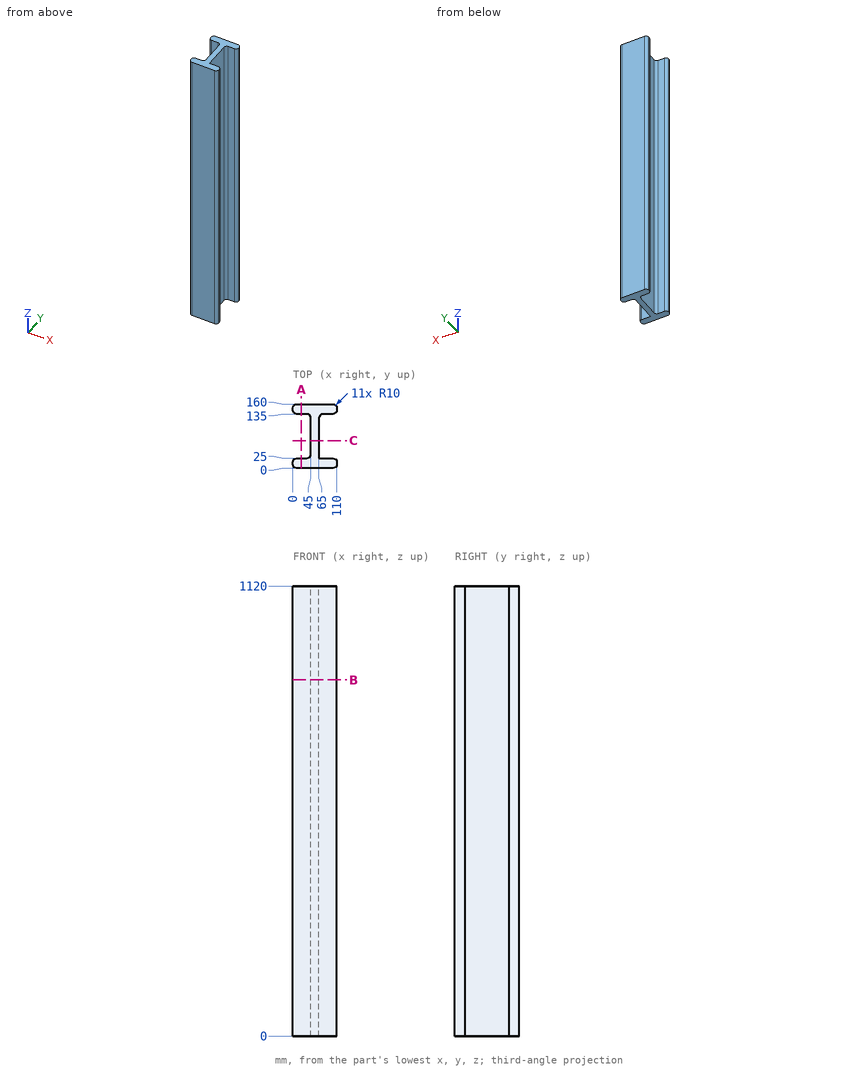
Geometry: see drawing. Coordinates: mm, zero at the bounding-box minimum. Coordinates: 2 decimals unless noted, no trailing zeros. Write each loop counter-clockwise with the first axis right and the second up, starting at its lowest first coordinate (ties: lowest second). Pieces come first, ordered by that corner, then holes. Notation, with made-up numbers: M 18,69 L 31,69 A17 cw 31,81 Z; hole C 11,50 d6. An arc over 180 degrees is marked long. Answer as a JSON object with one key per item and string values.
1. Cut plane C-C on y = 69. Output: boundary loops of the cut face in (x, z).
Evaluation:
{"outline": "M 45,0 L 65,0 L 65,1120 L 45,1120 Z"}
2. Ray query, L1, parallel to Y at x = 99, z = 923.5; L2, parallel to X at y = 111, z = 421.5; L3, parallel to X at y = 33.5, z = 608.5. Return the intervals inside material, ascending.
Evaluation:
{"L1": "0 to 25, 135 to 160", "L2": "45 to 65", "L3": "44.89 to 65"}
3. Cut plane A-A on x = 21.5. Output: boundary loops of the cut face in (y, z), plus the area to 3 significant figures.
Evaluation:
{"outline": "M 0,0 L 25,0 L 25,1120 L 0,1120 Z; M 135,0 L 160,0 L 160,1120 L 135,1120 Z", "area": "56,000 mm^2"}
4. Contact query for a flat-ended pin moving along its axis: P1, Ø6, axis at y = 83.5, z = 216.5, coming from the -X side. Output: stop coordinate, or through.
Evaluation:
{"P1": "x = 45"}
5. Cut plane B-B on z = 887. Output: boundary loops of the cut face in (x, y).
Evaluation:
{"outline": "M 0,10 A10 ccw 10,0 L 100,0 A10 ccw 110,10 L 110,15 A10 ccw 100,25 L 65,25 L 65,125 A10 cw 75,135 L 100,135 A10 ccw 110,145 L 110,150 A10 ccw 100,160 L 10,160 A10 ccw 0,150 L 0,145 A10 ccw 10,135 L 35,135 A10 cw 45,125 L 45,35 A10 cw 35,25 L 10,25 A10 ccw 0,15 Z"}
